Design review of the part built by this model. Coordinates are the model's own, in mm. A direction names the side the tool comes from. Give positions to 0.01 mm unless a question says otherwise; leave off trailing zeros. Write each loop counter-clockwise with the first axis right and the second up, starting at its lowest first coordinate (ties: lowest second). Pieces come first, ordered by that corner, then holes. Notation, with made-up numbers: M -24,72 L -13,72 A6 ccw -13,83 Z; hole C 64,-17 d5. An arc over 180 degrees is marked long. Use one line per item in the form item = value. Start each with the question number.
Autodesk Inventor part; units mm, degrees
ref_plane "YZ Plane" through (0, 0, 0) normal (1, 0, 0) x (0, 1, 0)
ref_plane "XZ Plane" through (0, 0, 0) normal (0, 1, 0) x (-1, 0, 0)
ref_plane "XY Plane" through (0, 0, 0) normal (0, 0, 1) x (1, 0, 0)
sketch "Sketch1" plane through (0, 0, 0) normal (0, 1, 0) x (-1, 0, 0)
  line L0 (33, 44) -> (-33, 44) construction
  line L1 (-33, 44) -> (-33, -44) construction
  line L2 (-33, -44) -> (33, -44) construction
  line L3 (33, -44) -> (33, 44) construction
  line L4 (33, 49) -> (-33, 49)
  line L5 (-38, 44) -> (-38, -44)
  line L6 (-33, -49) -> (33, -49)
  line L7 (38, -44) -> (38, 44)
  arc A0 (38, 44) -> (33, 49) centre (33, 44) ccw
  arc A1 (-33, 49) -> (-38, 44) centre (-33, 44) ccw
  arc A2 (-38, -44) -> (-33, -49) centre (-33, -44) ccw
  arc A3 (33, -49) -> (38, -44) centre (33, -44) ccw
  line L8 (-33, 47) -> (33, 47)
  arc A4 (36, 44) -> (33, 47) centre (33, 44) ccw
  line L9 (36, 44) -> (36, -44)
  arc A5 (33, -47) -> (36, -44) centre (33, -44) ccw
  line L10 (33, -47) -> (-33, -47)
  arc A6 (-36, -44) -> (-33, -47) centre (-33, -44) ccw
  line L11 (-36, -44) -> (-36, 44)
  arc A7 (-33, 47) -> (-36, 44) centre (-33, 44) ccw
  circle A8 centre (33, 44) radius 1.65
  circle A9 centre (33, -44) radius 1.65
  circle A10 centre (-33, -44) radius 1.65
  circle A11 centre (-33, 44) radius 1.65
  line L12 (33, 39) -> (28, 44)
  line L13 (28, 44) -> (-28, 44)
  line L14 (-28, 44) -> (-33, 39)
  line L15 (-33, 39) -> (-33, -39)
  line L16 (-33, -39) -> (-28, -44)
  line L17 (-28, -44) -> (28, -44)
  line L18 (28, -44) -> (33, -39)
  line L19 (33, -39) -> (33, 39)
  point P0 (0, 0)
  point P1 (33, 0)
  point P2 (38, 49)
  point P3 (-38, 49)
  point P4 (38, -49)
  point P5 (-38, 0)
  point P6 (0, 49)
  point P7 (0, 44)
  dimension "d0" = 76
  dimension "d1" = 98
  dimension "d2" = 5
  dimension "d3" = 2
  dimension "d4" = 3.3
  dimension "d5" = 1.35
  dimension "d6" = 1.35
  dimension "d7" = 66
  dimension "d8" = 88
  dimension "d9" = 5
  dimension "d10" = 3.5355
extrude "Extrusion1" add sketch "Sketch1" along normal mid plane 3.5 contours A0 L7 A3 L6 A2 L5 A1 L4 | L8 A4 L9 A5 L10 A6 L11 A7
fillet "Fillet1" radius 2 8 edges at (-33, 0, -39) (-28, 0, -44) (28, 0, -44) (33, 0, -39) (33, 0, 39) (28, 0, 44) (-33, 0, 39) (-28, 0, 44)
extrude "Extrusion2" cut sketch "Sketch1" along normal blind 1.25 and the other way blind 1.75 contours A0 L7 A3 L6 A2 L5 A1 L4
properties part number "SolarPanel_CoilForm" material "ABS Plastic"
1. We need section B-B (z = 35). State the section outline as (x, y) points.
2. To check wall thickness, follow L1, parallel to X at y = 1.5, z = 35.5; L2, parallel to X at y = 0.15, z = 20.5; L3, parallel to Z at x = 34.5, y = 1.65. State the ranges of each line that lie inside material, in increasing order.
3. Clearance check with flat-ended pins moving along their axes: pin 1 Ø1 at (x, y) = (-5.5, -1.5) entering from +Z; pin 2 Ø3 at (x, z) = (33, -44) entering from +Y; pin 3 Ø0.9 at (y, z) = (-0.5, 18) entering from +X; pin 4 Ø1 at (y, z) = (0, -12.5) entering from -X. State where each tip first meets the part, or that it passes through.
4. We need section A-A (x = 10.5). State the section outline as (y, z) points, and give its area (3 significant figures).
5. For faces 1 (the flat face through (0, 0, -47)), 2 (the flat face through (-33, 0, -1)), 3 (the flat face through (36, 0, -1)), list the 3-axis set-ups (+Z, -Z, +X, -X, +Y, -Y) from which the entire face can be reached by the end or side of a thin tool; tool diameter is ignored.
6. We need section C-C (y = -0.2). State the section outline as (x, z) points, and give its area (3 significant figures).
Answer block:
q1.outline = M -38,1.25 L -36,1.25 L -36,-1.75 L -33,-1.75 L -33,1.75 L -38,1.75 Z; M 33,-1.75 L 36,-1.75 L 36,1.25 L 38,1.25 L 38,1.75 L 33,1.75 Z
q2.L1 = -38 to -33, 33 to 38
q2.L2 = -36 to -33, 33 to 36
q2.L3 = -48.77 to -44.69, -43.31 to 43.31, 44.69 to 48.77
q3.pin_1 = 47
q3.pin_2 = through
q3.pin_3 = 36
q3.pin_4 = -36
q4.outline = M -1.75,-47 L 1.25,-47 L 1.25,-49 L 1.75,-49 L 1.75,-44 L -1.75,-44 Z; M -1.75,44 L 1.75,44 L 1.75,49 L 1.25,49 L 1.25,47 L -1.75,47 Z
q4.area = 23.0 mm^2
q5.face_1 = -Z, +X, -X, -Y
q5.face_2 = +Y, -Y
q5.face_3 = +Z, -Z, +X, -Y
q6.outline = M -36,-44 A3 ccw -33,-47 L 33,-47 A3 ccw 36,-44 L 36,44 A3 ccw 33,47 L -33,47 A3 ccw -36,44 Z; hole C -33,-44 d3.3; hole C -33,44 d3.3; hole M -33,-38.17 A2 ccw -32.41,-39.59 L -28.59,-43.41 A2 ccw -27.17,-44 L 27.17,-44 A2 ccw 28.59,-43.41 L 32.41,-39.59 A2 ccw 33,-38.17 L 33,38.17 A2 ccw 32.41,39.59 L 28.59,43.41 A2 ccw 27.17,44 L -27.17,44 A2 ccw -28.59,43.41 L -32.41,39.59 A2 ccw -33,38.17 Z; hole C 33,-44 d3.3; hole C 33,44 d3.3
q6.area = 969 mm^2
